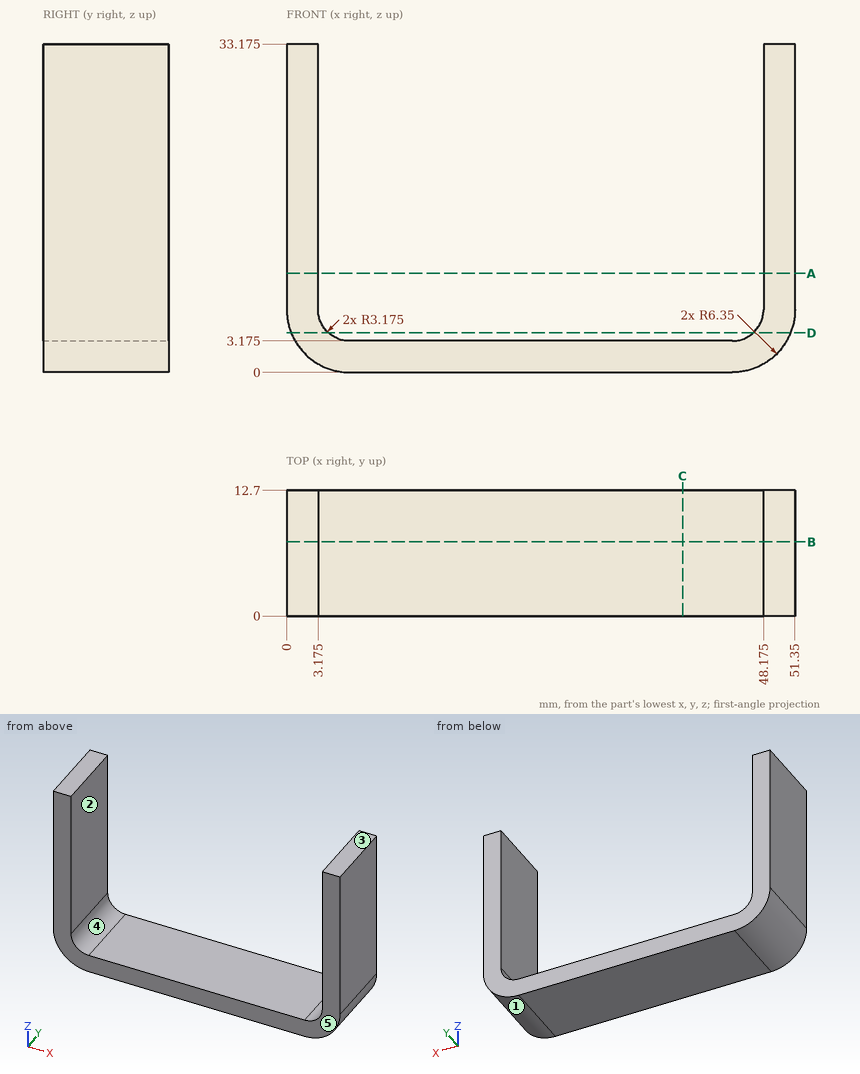
Source: three-view drawing plus pictorial views. Frame: mm from the lowest corner of the part. A direction names the side the tool comes from. Coordinates: 2 decimals unless noted, no trailing zeros. Loops run counter-clockwise (first coordinate to the right, second up) from the corner with the lowest first, then second, coordinate; pieces in that order, holes last. Notation, with made-up numbers: (-5.5, 50) - (40.5, 50) arc R5 cw to (40.5, 57) - close; hole circle Ø2 at (75.25, -11). An arc over 180 degrees is marked (long way). One line per item, written item: value. Start each with the question number.
1. Mould query, pull axis X, two halves, no side actions, for the marked faces 1, 2 and 3. Classes: pulls with the +X half, pulls with the -X half, needs draft (parallel to the pull), parting line crosses it, or undercut.
2. Set-up query: the marked faces 4 and 5. Return all of +Z, -Z, +X, -X, +Y, -Y with unobstructed straight access to the full face (end or side cutting, diameter ignored); none if empty.
3. Section C-C (x = 40). Return the cut outline in (y, z) (3 decimals).
4. Section A-A (z = 10). Return the cut outline in (x, y) (3 decimals), and give its area (3 significant figures).
5. Section D-D (z = 4). Return the cut outline in (x, y).
6. Ray query, L1, parallel to X at y = 2, z = 30 (3 decimals); L2, parallel to Z at x = 22, y = 6.75 (3 decimals); L3, parallel to X at y = 9.5, z = 3.5. Return the intervals inside material, ascending.
7. Contact query for flat-ended pins moving along their axis: P1, Ø5, axis at x = 6, y = 3.5, coming from the +Z side; P2, Ø4, axis at x = 17, y = 5.5, coming from the +Z side (3 decimals). Output: stop coordinate, or through.
8. Section B-B (y = 7.5). Return the cut outline in (x, z) (3 decimals).
Verdict:
1. face 1: pulls with the +X half
1. face 2: undercut
1. face 3: needs draft
2. face 4: +Z, +Y, -Y
2. face 5: +Z, -Z, +X, -X, -Y
3. outline: (0, 0) - (12.7, 0) - (12.7, 3.175) - (0, 3.175) - close
4. outline: (0, 0) - (3.175, 0) - (3.175, 12.7) - (0, 12.7) - close; (48.175, 0) - (51.35, 0) - (51.35, 12.7) - (48.175, 12.7) - close
4. area: 80.6 mm2
5. outline: (0.45, 0) - (4.22, 0) - (4.22, 12.7) - (0.45, 12.7) - close; (47.13, 0) - (50.9, 0) - (50.9, 12.7) - (47.13, 12.7) - close
6. L1: x = 0 to 3.175, 48.175 to 51.35
6. L2: z = 0 to 3.175
6. L3: x = 0.68 to 4.95, 46.4 to 50.67
7. P1: stops at z = 4.95
7. P2: stops at z = 3.175
8. outline: (0, 6.35) arc R6.35 ccw to (6.35, 0) - (45, 0) arc R6.35 ccw to (51.35, 6.35) - (51.35, 33.175) - (48.175, 33.175) - (48.175, 6.35) arc R3.175 cw to (45, 3.175) - (6.35, 3.175) arc R3.175 cw to (3.175, 6.35) - (3.175, 33.175) - (0, 33.175) - close
